Autodesk Fusion 360 part; units mm, degrees
sketch "Sketch1" plane through (0, 0, 0) normal (0, 0, 1) x (1, 0, 0)
  line L0 (0, 0) -> (120, 0)
  line L1 (120, 0) -> (120, 10)
  line L2 (120, 10) -> (0, 10)
  line L3 (0, 10) -> (0, 0)
  dimension "d1" = 120
  dimension "d2" = 10
extrude "Extrude1" add sketch "Sketch1" along normal blind 60
sketch "Sketch2" plane through (0, 0, 0) normal (0, 0, -1) x (1, 0, 0)
  line L0 (0, 0) -> (0, -10)
  line L1 (0, -10) -> (120, -10)
  line L2 (120, -10) -> (120, 0)
  line L3 (120, 0) -> (0, 0)
  line L4 (0, -5) -> (120, -5) construction
  point P0 (10, -5)
  point P1 (110, -5)
  dimension "d5" = 100
  dimension "d6" = 10
sketch "Sketch3" plane through (0, 0, 60) normal (0, 0, 1) x (-1, 0, 0)
  line L0 (0, -10) -> (0, 0)
  line L1 (0, 0) -> (-120, 0)
  line L2 (-120, 0) -> (-120, -10)
  line L3 (-120, -10) -> (0, -10)
  line L4 (0, -5) -> (-120, -5) construction
  point P0 (-10, -5)
  point P1 (-110, -5)
  dimension "d10" = 100
  dimension "d11" = 10
hole "Hole2" at (10, 5, 0) at (110, 5, 0) direction (0, 0, 1) diameter 4 depth 6 tip angle 180
hole "Hole3" at (10, 5, 60) at (110, 5, 60) direction (0, 0, -1) diameter 4 depth 6 tip angle 180
sketch "Sketch8" plane through (0, 10, 0) normal (0, 1, 0) x (-1, 0, 0)
  line L0 (-120, 0) -> (0, 0)
  line L1 (0, 0) -> (0, 60)
  line L2 (0, 60) -> (-120, 60)
  line L3 (-120, 60) -> (-120, 0)
  circle A0 centre (-99, 56.5) radius 1.35
  circle A1 centre (-41, 56.5) radius 1.35
  circle A2 centre (-99, 7.5) radius 1.35
  circle A3 centre (-41, 7.5) radius 1.35
  point P0 (-99, 56.5)
  point P1 (-41, 56.5)
  point P2 (-41, 7.5)
  point P3 (-99, 7.5)
hole "Hole5" at (99, 10, 56.5) at (41, 10, 56.5) at (99, 10, 7.5) at (41, 10, 7.5) direction (0, -1, 0) diameter 3 end through all counterbore diameter 5 counterbore depth 8
sketch "Sketch9" plane through (0, 0, 0) normal (0, -1, 0) x (1, 0, 0)
  circle A0 centre (99, 7.5) radius 1.5
  circle A1 centre (99, 56.5) radius 1.5
  circle A2 centre (41, 56.5) radius 1.5
  circle A3 centre (41, 7.5) radius 1.5
  line L0 (0, 0) -> (120, 0)
  line L1 (120, 0) -> (120, 60)
  line L2 (120, 60) -> (0, 60)
  line L3 (0, 60) -> (0, 0)
  circle A4 centre (41, 7.5) radius 3
  circle A5 centre (99, 7.5) radius 3
  circle A6 centre (99, 56.5) radius 3
  circle A7 centre (41, 56.5) radius 3
  dimension "d33" = 6
  dimension "d34" = 6
  dimension "d35" = 6
  dimension "d36" = 6
extrude "Extrude4" add sketch "Sketch9" along normal blind 4 contours A4 | A5 | A6 | A7
sketch "Sketch10" plane through (0, 0, 0) normal (0, -1, 0) x (1, 0, 0)
  circle A0 centre (41, 56.5) radius 3
  circle A1 centre (99, 7.5) radius 3
  circle A2 centre (41, 7.5) radius 3
  circle A3 centre (99, 56.5) radius 3
  line L0 (0, 0) -> (120, 0)
  line L1 (120, 0) -> (120, 60)
  line L2 (120, 60) -> (0, 60)
  line L3 (0, 60) -> (0, 0)
  line L4 (20, 0) -> (20, 60)
  arc A4 (100, 14.933) -> (100, 0.067) centre (99, 7.5) ccw
  arc A5 (34.3668, 60) -> (47.6332, 60) centre (41, 56.5) ccw
  line L5 (20, 60) -> (34.3668, 60)
  line L6 (47.6332, 60) -> (92.3668, 60)
  line L7 (33.5, 7.5) -> (33.5, 0)
  line L8 (48.5, 7.5) -> (48.5, 0)
  arc A6 (48.5, 7.5) -> (33.5, 7.5) centre (41, 7.5) ccw
  line L9 (100, 0) -> (48.5, 0)
  line L10 (33.5, 0) -> (20, 0)
  line L11 (100, 60) -> (100, 14.933)
  line L12 (100, 10.3284) -> (100, 4.6716)
  line L13 (100, 0.067) -> (100, 0)
  arc A7 (92.3668, 60) -> (100, 49.067) centre (99, 56.5) ccw
  dimension "d39" = 15
  dimension "d40" = 15
  dimension "d41" = 15
  dimension "d42" = 15
  dimension "d43" = 20
  dimension "d44" = 20
extrude "Extrude5" cut sketch "Sketch10" against normal blind 5 contours L0 L2 L4 A4 A5 L5 L6 L7 L8 A6 L9 L10 L11 A7
equation "d6 = ( 120 mm - d5 ) / 2"
equation "d11 = ( 120 mm - d10 ) / 2"
equation "d34 = d33"
equation "d35 = d33"
equation "d36 = d33"
equation "d40 = d39"
equation "d41 = d39"
equation "d42 = d39"
CAD build for the part. Positions are in the model's coordinates, mm. A direction names the side the tool comes from. Coordinates: 2 decimals unless noted, no trailing zeros. Write each loop counter-clockwise with the first axis right and the second up, starting at its lowest first coordinate (ties: lowest second). Pieces come first, ordered by that corner, then holes. Notation, with made-up numbers: (73, -37.5) - (118, -37.5) arc R28 cw to (118, -14.5) - close; hole circle Ø7 at (16.5, 84). An arc over 180 degrees is marked (long way). Use a Markdown table: item, result. Add a question column.
Item 1: Band-saw the part on D-D, the plane x = 110. Give the cut face in (y, z), and give its area (3 significant figures).
Item 2: Drill centre lines: L1, parallel to Z at x = 99, y = -1.05; L2, parallel to X at y = 1.3, z = 7.5; L3, parallel to Y at x = 110, z = 56.1. Where is each one in solid material? Low to high. Write a range as from..to.
Item 3: Flat gauge pins, fed straight in: pin 1 (4 mm diameter, centred on x = 99, z = 56.5, fed in from +Y); pin 2 (18 mm diameter, centred on x = 43.5, z = 40.5, fed in from -Y). Where does each tip first touch, or does it go through?
Item 4: Band-saw the part on A-A, the plane x = 41. Give the number of separate pieces and of enclosed holes in the cut face, and give its area (3 significant figures).
Item 5: Mould opens along X. For faces 1 (the face through (59, 6, 0)), 2 (the face through (120, 5, 30)), 3 (the face through (100, 2, 32)) say: pulls with the +X half, pulls with the -X half, needs draft (parallel to the pull), parting line crosses it, or undercut.
Item 6: Band-saw the part on C-C, the plane z = 38. Give the cut face in (x, y), and give its area (3 significant figures).
Item 7: 3-axis set-ups, long thin cutter, end or side, ignore diameter. For faces 4 (the face through (41, 2, 15)), 5 (the face through (96.52, 5.94, 56.17)), 6 (the face through (108, 5, 3)), 7 (the face through (20, 2, 30)): which of +Z, -Z, +X, -X, +Y, -Y reach the whole face in a straight line?
Numbers:
| question | item | result |
|---|---|---|
| 1 | outline | (0, 0) - (3, 0) - (3, 6) - (7, 6) - (7, 0) - (10, 0) - (10, 60) - (7, 60) - (7, 54) - (3, 54) - (3, 60) - (0, 60) - close |
| 1 | area | 552 mm2 |
| 2 | L1 | 4.5..6, 9..10.5, 53.5..55, 58..59.5 |
| 2 | L2 | 0..20, 33.5..39.5, 42.5..48.5, 91.5..97.5, 100.5..120 |
| 2 | L3 | 0..3, 7..10 |
| 3 | pin 1 | y = 2 |
| 3 | pin 2 | y = 0 |
| 4 | separate pieces | 3 |
| 4 | enclosed holes | 0 |
| 4 | area | 362 mm2 |
| 5 | face 1 | needs draft |
| 5 | face 2 | pulls with the +X half |
| 5 | face 3 | undercut |
| 6 | outline | (0, 0) - (20, 0) - (20, 5) - (100, 5) - (100, 0) - (120, 0) - (120, 10) - (0, 10) - close |
| 6 | area | 800 mm2 |
| 7 | face 4 | -Y |
| 7 | face 5 | +Y |
| 7 | face 6 | -Z |
| 7 | face 7 | +Z, -Z, -Y |
